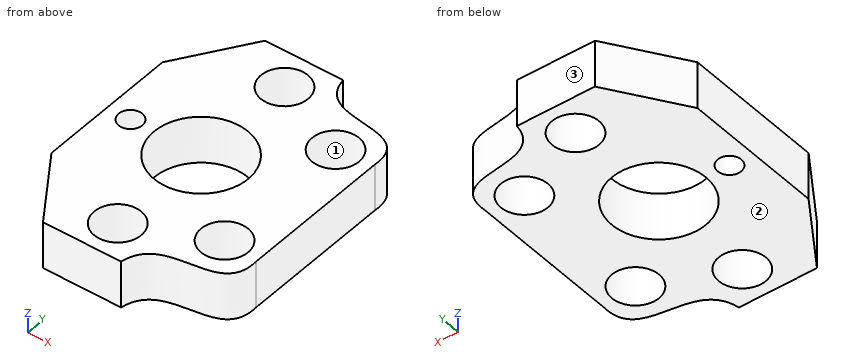
```python
from build123d import *

# Parameters (mm, degrees)
SKETCH1_R           = 10
SKETCH1_R_2         = 2.5
SKETCH1_R_3         = 5
BOSS_EXTRUDE1_DEPTH = 10


with BuildPart() as part:
    # Sketch1 → Boss-Extrude1 (new body)
    with BuildSketch(Plane.XY):
        with BuildLine():
            Line((-20, -22.406552459), (-20, 7.593447541))
            Line((-20, 7.593447541), (-10, 22.593447541))
            Line((-10, 22.593447541), (0, 22.593447541))
            Line((0, 22.593447541), (6.589653899, 22.593447541))
            add(Edge.make_bspline(
                [(6.589653899, 22.593447541), (8.279830639, 11.435624487), (25.165546695, 20.477646142), (24.304134066, 8.692145069)],
                knots=[0, 0, 0, 0, 1, 1, 1, 1], degree=3))
            Line((24.304134066, 8.692145069), (24.304134066, -23.505249987))
            add(Edge.make_bspline(
                [(6.589653899, -37.406552459), (8.279830639, -26.248729405), (25.165546695, -35.290751061), (24.304134066, -23.505249987)],
                knots=[0, 0, 0, 0, 1, 1, 1, 1], degree=3))
            Line((6.589653899, -37.406552459), (0, -37.406552459))
            Line((0, -37.406552459), (-10, -37.406552459))
            Line((-10, -37.406552459), (-20, -22.406552459))
        make_face()
        with Locations(Location((0, -7.406552459, 0), (0, 0, 180))):
            Circle(SKETCH1_R, mode=Mode.SUBTRACT)
        with Locations((-15, -7.406552459)):
            Circle(SKETCH1_R_2, mode=Mode.SUBTRACT)
        with Locations((0, 15.12355642)):
            Circle(SKETCH1_R_3, mode=Mode.SUBTRACT)
        with Locations((16.779399128, 7.593447541)):
            Circle(SKETCH1_R_3, mode=Mode.SUBTRACT)
        with Locations(Location((0, -29.936661338, 0), (0, 0, 180))):
            Circle(SKETCH1_R_3, mode=Mode.SUBTRACT)
        with Locations(Location((16.779399128, -22.406552459, 0), (0, 0, 180))):
            Circle(SKETCH1_R_3, mode=Mode.SUBTRACT)
    extrude(amount=BOSS_EXTRUDE1_DEPTH)


solid = part.part
```
Input: part model. Units: mm. Frame: model coordinates. Face numbers are marked on the shaded views. Round coordinates to 2 decimals unless told otherwise and drop trailing zeros. Loops run counter-clockwise (first coordinate to the right, second up) from the corner with the lowest first, then second, coordinate; pieces in that order, holes last. Notation, with made-up numbers: M 18.5,31.25 L 63.5,31.25 A8 ccw 63.5,35.25 Z; hole C 41,-15.75 d11. An arc over 180 degrees is marked long. Answer in a Markdown table with one row per item. Add a question column.
1. Mould query, pull axis Y, two halves, no side actions, for the marked faces 1, 2 and 3. Classes: released by +Y, released by -Y, zero draft, split by the parting line, or undercut.
2. Section C-C (x = -14). Output: boundary loops of the cut face in (y, z), and give its area (3 significant figures).
3. Section D-D (z = 2.25). Give the number of separate pieces and of enclosed holes in the cut face, and give its area (3 significant figures).
4. Contact query for a flat-ended pin moving along its axis: pin 1 (5 mm diameter, centred on y = -1.5, z = 6, fed in from +X). Output: stop coordinate, or through.
5. Section A-A (x = 0). Output: boundary loops of the cut face in (y, z).
6. Ray query, probe 1 along Y at (x, z) = (0, 3.25); probe 2 along Y at (x, z) = (19, 1); probe 3 along Y at (x, z) = (21, 5). Return the intervals inside material, ascending.
7. Section B-B (y = -3.5). Output: boundary loops of the cut face in (x, z), and give its area (3 significant figures).
Values follow:
| question | item | result |
|---|---|---|
| 1 | face 1 | undercut |
| 1 | face 2 | zero draft |
| 1 | face 3 | released by +Y |
| 2 | outline | M -31.41,0 L -9.7,0 L -9.7,10 L -31.41,10 Z; M -5.12,0 L 16.59,0 L 16.59,10 L -5.12,10 Z |
| 2 | area | 434 mm^2 |
| 3 | separate pieces | 1 |
| 3 | enclosed holes | 6 |
| 3 | area | 1,630 mm^2 |
| 4 | pin 1 | x = 24.3 |
| 5 | outline | M -37.41,0 L -34.94,0 L -34.94,10 L -37.41,10 Z; M -24.94,0 L -17.41,0 L -17.41,10 L -24.94,10 Z; M 2.59,0 L 10.12,0 L 10.12,10 L 2.59,10 Z; M 20.12,0 L 22.59,0 L 22.59,10 L 20.12,10 Z |
| 6 | probe 1 | -37.41 to -34.94, -24.94 to -17.41, 2.59 to 10.12, 20.12 to 22.59 |
| 6 | probe 2 | -30.26 to -26.89, -17.93 to 3.11, 12.07 to 15.45 |
| 6 | probe 3 | -29.67 to -25.09, -19.73 to 4.91, 10.27 to 14.86 |
| 7 | outline | M -20,0 L -9.21,0 L -9.21,10 L -20,10 Z; M 9.21,0 L 24.3,0 L 24.3,10 L 9.21,10 Z |
| 7 | area | 259 mm^2 |
